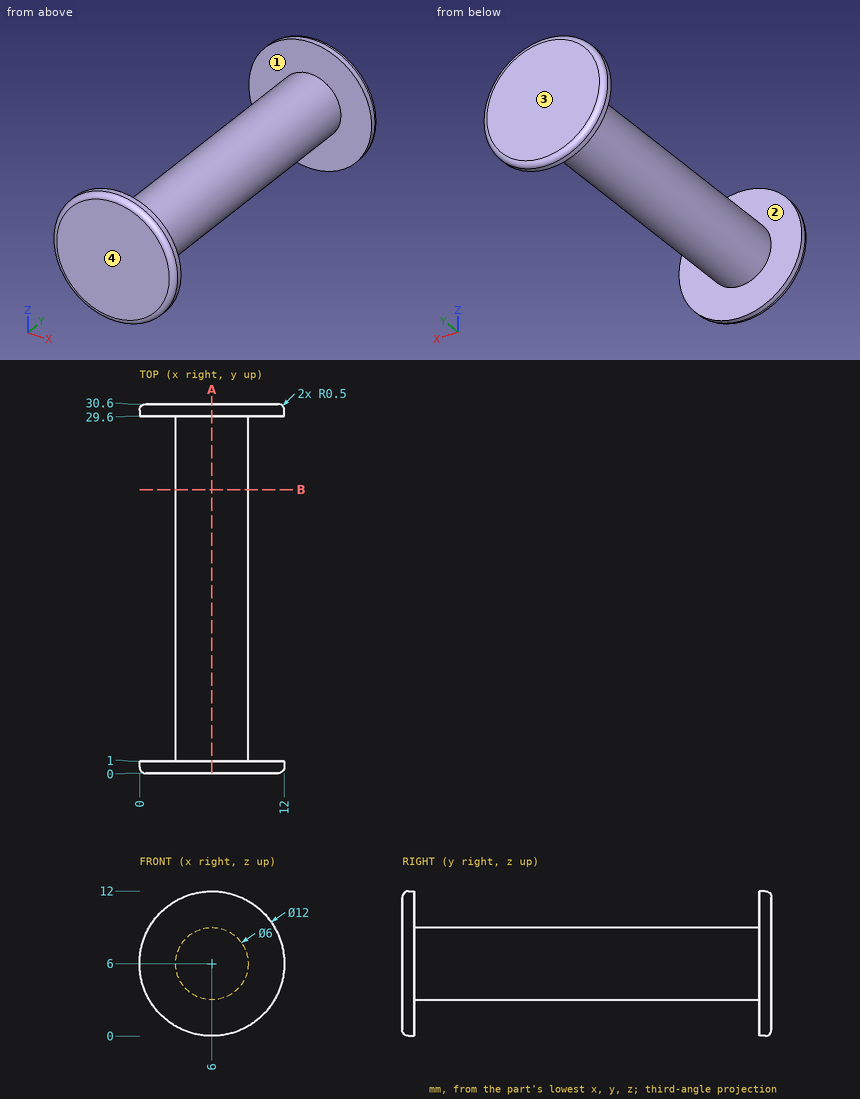
Geometry: see drawing. Coordinates: mm, zero at the bounding-box minimum. Give positions to 0.01 mm unless a question says otherwise; leave off trailing zeros. Order: outer loops, then holes, each group sorted by start corner. A loop starts at its lowest first (then second) coordinate and runs counter-clockwise, first axis right, second up. Notation, with made-up numbers: (10.5, 37.25) - (15.5, 37.25) arc R34 cw to (15.5, 74.25) - close; hole circle Ø1 at (63.25, 39). An arc over 180 degrees is marked (long way). Use CSV: the item, a comma, the result in double quotes.
1. Contact query for flat-ended pins moving along their axis: pin 1 (2 mm diameter, centred on x = 2, z = 10.5, fed in from +Y); pin 2 (4 mm diameter, centred on y = 11, z = 8, fed in from -X); pin 3 (2 mm diameter, centred on y = 7, z = 5.5, fed in from +X); pin 4 (5 mm diameter, centred on y = 19.5, z = 10, fed in from -X). Output: stop coordinate, or through.
Answers below:
pin 1,"y = 30.6"
pin 2,"x = 3"
pin 3,"x = 9"
pin 4,"x = 3.4"
2. Section query A-A (x = 6). Output: boundary loops of the cut face in (y, z).
Answers below:
outline,"(0, 0.5) arc R0.5 ccw to (0.5, 0) - (1, 0) - (1, 3) - (29.6, 3) - (29.6, 0) - (30.1, 0) arc R0.5 ccw to (30.6, 0.5) - (30.6, 11.5) arc R0.5 ccw to (30.1, 12) - (29.6, 12) - (29.6, 9) - (1, 9) - (1, 12) - (0.5, 12) arc R0.5 ccw to (0, 11.5) - close"
3. Mould query, pull axis Y, two halves, no side actions, for the marked faces 1, 2, 3 and 4. Classes: +Y half, -Y half, draft (parallel to the pull), parting line (faces both ways), or undercut.
Answers below:
face 1,"undercut"
face 2,"undercut"
face 3,"+Y half"
face 4,"-Y half"
4. Material intervals for line 1 along Y through (x, z) = (7.75, 10.5); line 2 along Y through (x, z) = (2, 1.75); line 3 along X through (y, z) = (5, 4.75), sorted ascending. Write a range as from..to.
Answers below:
line 1,"0..1, 29.6..30.6"
line 2,"0.13..1, 29.6..30.47"
line 3,"3.27..8.73"
5. Section query B-B (y = 23.5). Output: boundary loops of the cut face in (x, z), plus the area to 3 significant figures.
Answers below:
outline,"circle Ø6 at (6, 6)"
area,"28.3 mm2"
